Read the model definition and answer for the solid it produces. Units are mm, in the model's axes. A direction names the side the tool comes from. Coordinates: 2 decimals unless noted, no trailing zeros. Order: outer loops, then holes, each group sorted by start corner. A loop starts at its lowest first (then second) coordinate and runs counter-clockwise, first axis right, second up.
from build123d import *

# Parameters (mm, degrees)
SKETCH6_W           = 140
SKETCH6_H           = 40
BOSS_EXTRUDE2_DEPTH = 30
SKETCH9_W           = 7
SKETCH9_H           = 40
CUT_EXTRUDE3_DEPTH  = 40
CUT_EXTRUDE6_DEPTH  = 45
CUT_EXTRUDE7_DEPTH  = 45
SKETCH22_R          = 4.1
CUT_EXTRUDE8_DEPTH  = 45
CUT_EXTRUDE9_DEPTH  = 45
SKETCH26_R          = 10
CUT_EXTRUDE10_DEPTH = 10
SKETCH28_R          = 5
CUT_EXTRUDE11_DEPTH = 35


with BuildPart() as part:
    # Sketch6 → Boss-Extrude2 (new body)
    with BuildSketch(Plane(origin=(0, 0, 0), x_dir=(0, 0, -1), z_dir=(1, 0, 0))):
        Rectangle(SKETCH6_W, SKETCH6_H)
    extrude(amount=BOSS_EXTRUDE2_DEPTH)

    # Sketch9 → Cut-Extrude3 (cut)
    with BuildSketch(Plane.XY.offset(70)):
        with Locations((3.5, 0)):
            Rectangle(SKETCH9_W, SKETCH9_H)
        with Locations((26.5, 0)):
            Rectangle(SKETCH9_W, SKETCH9_H)
    extrude(amount=-CUT_EXTRUDE3_DEPTH, mode=Mode.SUBTRACT)

    # Sketch18 → Cut-Extrude6 (cut)
    with BuildSketch(Plane(origin=(23, 0, 0), x_dir=(0, 0, -1), z_dir=(1, 0, 0))):
        with BuildLine():
            Line((-70, 20), (-70, 0))
            ThreePointArc((-70, 0), (-64.142135624, 14.142135624), (-50, 20))
            Line((-50, 20), (-70, 20))
        make_face()
    extrude(amount=-CUT_EXTRUDE6_DEPTH, mode=Mode.SUBTRACT)

    # Sketch19 → Cut-Extrude7 (cut)
    with BuildSketch(Plane(origin=(23, 0, 0), x_dir=(0, 0, -1), z_dir=(1, 0, 0))):
        with BuildLine():
            Line((-70, 0), (-70, -20))
            Line((-70, -20), (-50, -20))
            ThreePointArc((-50, -20), (-64.142135624, -14.142135624), (-70, 0))
        make_face()
    extrude(amount=-CUT_EXTRUDE7_DEPTH, mode=Mode.SUBTRACT)

    # Sketch22 → Cut-Extrude8 (cut)
    with BuildSketch(Plane(origin=(23, 0, 0), x_dir=(0, 0, -1), z_dir=(1, 0, 0))):
        with Locations(Location((-50, 0, 0), (0, 0, 90))):
            Circle(SKETCH22_R)
    extrude(amount=-CUT_EXTRUDE8_DEPTH, mode=Mode.SUBTRACT)

    # Sketch24 → Cut-Extrude9 (cut)
    with BuildSketch(Plane(origin=(30, 0, 0), x_dir=(0, 0, -1), z_dir=(1, 0, 0))):
        Polygon((70, 20), (30, -20), (70, -20), align=None)
    extrude(amount=-CUT_EXTRUDE9_DEPTH, mode=Mode.SUBTRACT)

    # Sketch26 → Cut-Extrude10 (cut)
    with BuildSketch(Plane(origin=(0, -25, -25), x_dir=(1, 0, 0), z_dir=(0, -0.707106781186551, -0.7071067811865441))):
        with Locations(Location((15, -35.355339059, 0), (0, 0, 270))):
            Circle(SKETCH26_R)
    extrude(amount=-CUT_EXTRUDE10_DEPTH, mode=Mode.SUBTRACT)

    # Sketch28 → Cut-Extrude11 (cut)
    with BuildSketch(Plane(origin=(0, -17.928932188, -17.928932188), x_dir=(1, 0, 0), z_dir=(0, -0.7071067811865509, -0.7071067811865442))):
        with Locations(Location((15, -35.355339059, 0), (0, 0, 270))):
            Circle(SKETCH28_R)
    extrude(amount=-CUT_EXTRUDE11_DEPTH, mode=Mode.SUBTRACT)


solid = part.part
Q1. Each of these flat-tipped pins is pushed along its axis until it touches: P1, Ø8, axis at x = 11.5, y = 4, coming from the -Z side; P2, Ø8, axis at x = 4, y = 9, coming from the -Z side; P3, Ø2, axis at x = 28, y = -3.5, coming from the +Z side. Where does it stop, or does it pass through?
Q2. Which of the six approach directions +Z, -Z, +X, -X, +Y, -Y give full straight-line access (tool end or side, diameter ignored) to faces 4 (the flat face through (26, 0, 30)), 5 (the flat face through (7, 4, 46)), 6 (the flat face through (19.58, 5.4, -41.26))?
Q3. The part is cut by section B-B, the plane z = -60.5. Determine the outline of the cut face in (x, y).
Q4. Determine the mould class of faces 1 (the flat face through (25.2, 0.3, -50.3)), 2 (the cylindrical face through (15.22, 9.882, -33.053)), 3 (the flat face through (23, 4, 46)) for opening direction X: +X half, -X half, draft (parallel to the pull), parting line (faces both ways), or undercut.
Q5. Straight lines are drawn through the part: L1, parallel to Z at x = 14.5, y = 0; L2, parallel to X at y = 2.5, z = -47.5; L3, parallel to Z at x = 17.75, y = 0. For each, find the intervals that lie inside material, in ascending order.
Q6. The part is cut by section A-A, the plane x = 17. Determine the outline of the cut face in (y, z).
Computed values:
1. P1: stops at z = -58
1. P2: stops at z = -63
1. P3: stops at z = 30
2. face 4: +Z, +X, +Y, -Y
2. face 5: +Z, -X, +Y, -Y
2. face 6: none
3. outline: (0, 10.5) - (30, 10.5) - (30, 20) - (0, 20) - close
4. face 1: draft
4. face 2: undercut
4. face 3: +X half
5. L1: z = -35.88 to 45.9, 54.1 to 70
5. L2: x = 0 to 5, 25 to 30
5. L3: z = -36.4 to 45.9, 54.1 to 70
6. outline: (-20, -30) - (-6.93, -43.07) - (0.14, -36) - (3.83, -39.69) - (20, -23.52) - (20, 50) arc R20 ccw to (-20, 50) - close; (6.93, -56.93) - (20, -70) - (20, -36.48) - (10.31, -46.17) - (14, -49.86) - close; hole circle Ø8.2 at (0, 50)
